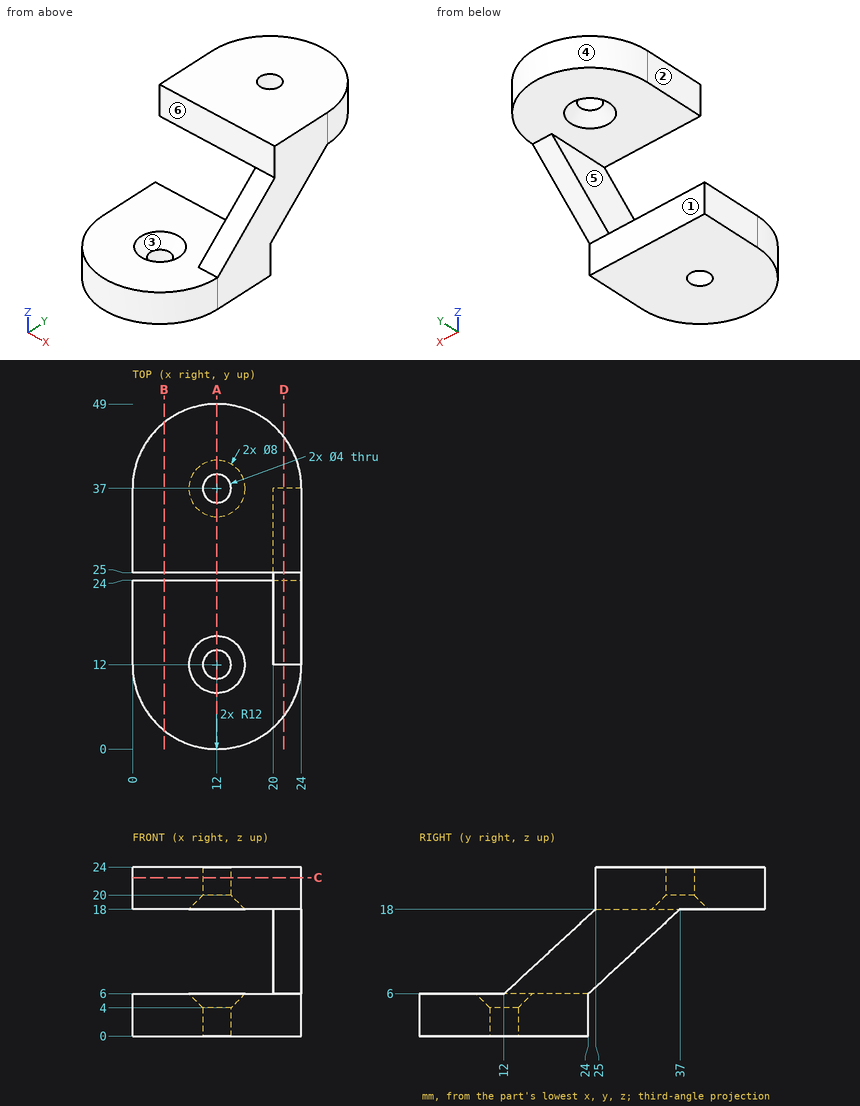
Drawing for the job (mm, zero at the part's lowest x, y, z). A direction names the side the tool comes from. Give positions to 0.01 mm unless a question says otherwise; leave off trailing zeros. Write each loop counter-clockwise with the first axis right and the second up, starting at its lowest first coordinate (ties: lowest second). Pieces come first, ordered by that corner, then holes. Notation, with made-up numbers: (50.25, 69.5) -> (61.25, 69.5) arc R27 cw to (61.25, 92.5) -> close; hole circle Ø4 at (40, 10). An arc over 180 degrees is marked (long way). Put each result on its own line as item: value. Start each with the question number.
Item 1: Which spindle directions (+Z, -Z, +X, -X, +Y, -Y) get a long thin tool onto all of the face, cutting with end or side? Do the marked faces 4, 5 and 6. Say none if no direction does.
Item 2: Pull direction X, two halves, no side cores. Call the marked faces 1, 2 and 3: pulls with the +X half, pulls with the -X half, needs draft (parallel to the pull), parting line crosses it, or undercut.
Item 3: Cut at C-C (z = 22.5). List the corners of the cut face in (x, y), then the cut area to 3 significant figures.
Item 4: Cut at B-B (x = 4.5). List the corners of the cut face in (y, z), then the cut area to 3 significant figures.
Item 5: Wall check: L1, parallel to Y at x = 12, z = 1.45; L2, parallel to Y at x = 12, z = 21.3; L3, parallel to Z at x = 13.25, y = 33. Give the ranges that are in metal, low to high. Write a range as [from, to].
Item 6: Cut at A-A (x = 12). List the corners of the cut face in (y, z), then the cut area to 3 significant figures.
Item 7: Cut at D-D (x = 21.5). List the corners of the cut face in (y, z), then the cut area to 3 significant figures.
Item 8: Pin check, flat tips, straight feed: pin 1 Ø4 at (y, z) = (27, 6.5) entering from +X; pin 2 Ø12 at (x, y) = (13, 31.5) entering from -Z; pin 3 Ø1.8 at (x, z) = (6, 3.5) entering from +Y; pin 4 Ø3 at (x, z) = (3, 20.5) entering from -Y. Stop position of each tip, or through.
Answer list:
1. face 4: +Z, -Z, +Y
1. face 5: -X, +Y, -Y
1. face 6: +Z, +X, -X, -Y
2. face 1: needs draft
2. face 2: pulls with the -X half
2. face 3: undercut
3. outline: (0, 25) -> (24, 25) -> (24, 37) arc R12 ccw to (0, 37) -> close; hole circle Ø4 at (12, 37)
3. area: 502 mm2
4. outline: (2.63, 0) -> (24, 0) -> (24, 6) -> (2.63, 6) -> close; (25, 18) -> (46.37, 18) -> (46.37, 24) -> (25, 24) -> close
4. area: 256 mm2
5. L1: y = [0, 10], [14, 24]
5. L2: y = [25, 35], [39, 49]
5. L3: z = [18, 24]
6. outline: (0, 0) -> (10, 0) -> (10, 4) -> (8, 6) -> (0, 6) -> close; (14, 0) -> (24, 0) -> (24, 6) -> (16, 6) -> (14, 4) -> close; (25, 18) -> (33, 18) -> (35, 20) -> (35, 24) -> (25, 24) -> close; (39, 20) -> (41, 18) -> (49, 18) -> (49, 24) -> (39, 24) -> close
6. area: 232 mm2
7. outline: (4.67, 0) -> (24, 0) -> (24, 6) -> (37, 18) -> (44.33, 18) -> (44.33, 24) -> (25, 24) -> (25, 18) -> (12, 6) -> (4.67, 6) -> close
7. area: 376 mm2
8. pin 1: stops at x = 24
8. pin 2: stops at z = 18
8. pin 3: stops at y = 24
8. pin 4: stops at y = 25
